For this review, take the finished solid that the model builds, in its own axes (mm). Round coordinates to 2 decimals unless told otherwise and drop trailing zeros. Write each loop counter-clockwise with the first axis right and the second up, starting at its lowest first coordinate (ties: lowest second). Pieces come first, ordered by that corner, then holes. Notation, with made-up numbers: M 73,25 L 104,25 A16 cw 104,45 Z; hole C 76,87.5 d9. An arc over 180 degrees is marked long. Write each question's results on one line, items separated by ' | '. Start each with the question number.
```python
from build123d import *

# Parameters (mm, degrees)
EXTRUDE_1_DEPTH = 6


with BuildPart() as part:
    # Эскиз1 → Бобышка-Вытянуть1 (new body)
    with BuildSketch(Plane(origin=(0, 0, 0), x_dir=(-1, 0, 0), z_dir=(0, 0, -1))):
        with BuildLine():
            Line((-265.446108594, 218.715019647), (3.734050958, 4.696473511))
            ThreePointArc((3.734050958, 4.696473511), (4.696473511, -3.734050958), (-3.734050958, -4.696473511))
            Line((-3.734050958, -4.696473511), (-130, 95.694487269))
            Line((-130, 95.694487269), (-130.871278557, 94.598643449))
            Line((-130.871278557, 94.598643449), (-4.605329515, -5.79231733))
            ThreePointArc((-4.605329515, -5.79231733), (5.79231733, -4.605329515), (4.605329515, 5.79231733))
            Line((4.605329515, 5.79231733), (-264.574830037, 219.810863466))
            ThreePointArc((-264.574830037, 219.810863466), (-274.972476883, 218.623875651), (-273.785489068, 208.226228806))
            Line((-273.785489068, 208.226228806), (-158.550793978, 116.60594762))
            Line((-158.550793978, 116.60594762), (-157.679515421, 117.70179144))
            Line((-157.679515421, 117.70179144), (-272.914210511, 209.322072625))
            ThreePointArc((-272.914210511, 209.322072625), (-273.876633064, 217.752597094), (-265.446108594, 218.715019647))
        make_face()
    extrude(amount=-EXTRUDE_1_DEPTH)


solid = part.part
```
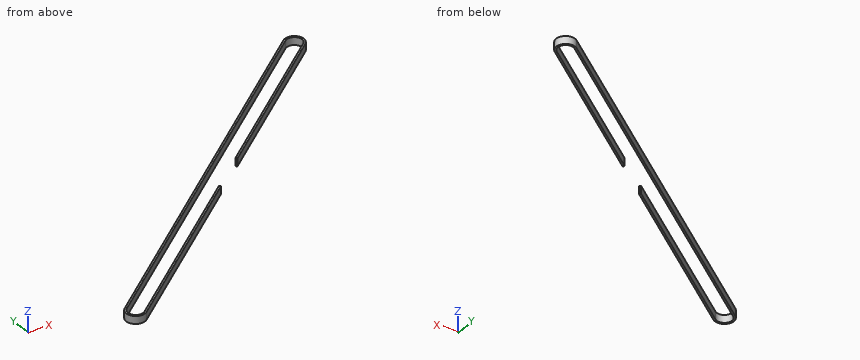
Item 1: Insertion check: P1, Ø1.5, axis at y = 60, z = 2, coming from the -X side; P2, Ø1.5, axis at x = 104, z = 2, coming from the +Y side. Each pin has a flat end and moves straight along its axis. Give the tip position at first contact, or say it passes through.
Item 2: We need section D-D on x = 147.5. State the section outline as (y, z) points, then the cut area to 3 significant figures.
Item 3: We need section B-B on x = 0. State the section outline as (y, z) points, then the cut area to 3 significant figures.
Item 4: We need section A-A on z = 1.35. State the section outline as (x, y) points, then the cut area to 3 significant figures.
Item 5: We need section C-C on y = 0. State the section outline as (x, z) points.
Item 6: For probe 1 along X at (y, z) = (210, 4.7); probe 2 along X at (y, z) = (194, 1.5); probe 3 along Y at (x, z) = (243, 3.5), list the stretches that pass through material, from the lowest coordinate up.
Numbers:
1) P1: stops at x = 62.63 | P2: stops at y = 92.74
2) outline: M 124.94,0 L 126.73,0 L 126.73,6 L 124.94,6 Z | area: 10.7 mm^2
3) outline: M -7.4,0 L -6,0 L -6,6 L -7.4,6 Z; M 7.67,0 L 9.45,0 L 9.45,6 L 7.67,6 Z | area: 19.1 mm^2
4) outline: M -4.61,5.79 A7.4 ccw 4.61,-5.79 L 130.87,94.6 L 130,95.69 L 3.73,-4.7 A6 cw -3.73,4.7 L 265.45,218.72 A6 cw 272.91,209.32 L 157.68,117.7 L 158.55,116.61 L 273.79,208.23 A7.4 ccw 264.57,219.81 Z | area: 972 mm^2
5) outline: M -7.4,0 L -6,0 L -6,6 L -7.4,6 Z; M 9.64,0 L 11.89,0 L 11.89,6 L 9.64,6 Z
6) probe 1: x = 252.24 to 254.48, 273.64 to 275.39 | probe 2: x = 232.11 to 234.36, 253.64 to 255.89 | probe 3: y = 183.75 to 185.54, 200.87 to 202.66
